Could you check a few things on this model? Use its own coordinates, in mm. A direction names the side the tool comes from. Round coordinates to 2 decimals unless told otherwise and drop trailing zeros. Write each loop counter-clockwise with the first axis right and the second up, starting at its lowest first coordinate (ties: lowest second). Pieces come first, ordered by that corner, then holes. Notation, with made-up numbers: (-31, -19) -> (-10, -19) arc R5 ccw to (-10, -15) -> close; hole circle Ø10 at (-38.75, 9). An arc over 180 degrees is marked (long way). Answer as CSV lines item,"result". Start each with the question number.
Q1. If we mould it in two halves opening along Z, with no side actions, what happens to faces 5 (the flat face through (42.99, -4.83, -6.68)), 6 (the cylindrical face through (8.33, 2.18, 22.03)), 7 (the flat face through (20.1, 3, 0))? For each: pulls with the +Z half, pulls with the -Z half, needs draft (parallel to the pull), parting line crosses it, or undercut.
Q2. Will these pins go through, and if not, where does the flat tip stop? pin 1 Ø3.5 at (x, y) = (8.9, 4) entering from -Z; pin 2 Ø3 at (x, z) = (55.5, 9) entering from +Y; pin 3 Ø3 at (y, z) = (21.51, 23.7) entering from -X.
Q3. Imagine slicing it at B-B on z = -16. Please give me the cut outline in (x, y), and give its area (3 significant figures).
Q4. Imagine slicing it at D-D on z = 35.2. Please give me the cut outline in (x, y).
Q5. Imagine slicing it at A-A on x = -5.6. Please give me the cut outline in (y, z).
Q6. For faces 1 (the flat face through (52.07, -2.02, 25.92)), 2 (the flat face through (0, 3, 20.1)), 3 (the cylindrical face through (71.44, -1.43, 25.05)), 4 (the flat face through (-23.9, 3, 0)), which set-ups out of +Z, -Z, +X, -X, +Y, -Y let a thin tool reach every point of the face, with its end or its side?
Q7. Imagine slicing it at C-C on y = 16.5. Please give me the cut outline in (x, z).
Q8. If I drill on line 1 (Y direction, x = 71, z = 46.7); line 2 (X direction, y = 2.5, z = 23); line 3 (Z direction, x = 20, y = 3.5), over which ranges is the centre line in solid material (lowest first)? Write a range as [from, to].
from build123d import *

# Parameters (mm, degrees)
SKETCH1_W            = 47.8
SKETCH1_H            = 47.8
SKETCH1_W_2          = 40.2
SKETCH1_H_2          = 40.2
BOSS_EXTRUDE1_DEPTH  = 6
CUT_EXTRUDE4_REACH   = 55.778
SKETCH6_R            = 1.35
CUT_EXTRUDE5_REACH   = 55.778
SKETCH7_R            = 1.35
SKETCH8_R            = 1.35
CUT_EXTRUDE6_DEPTH   = 54.777783517
SKETCH11_W           = 5
SKETCH11_H           = 28
SKETCH11_W_2         = 47.8
SKETCH11_H_2         = 47.8
SKETCH11_R           = 1.65
BOSS_EXTRUDE8_DEPTH  = 8
CUT_EXTRUDE7_DEPTH   = 105.25363303
SKETCH12_W           = 28
SKETCH12_H           = 28
SKETCH12_R           = 11.15
SKETCH12_R_2         = 1.35
SKETCH12_R_3         = 8.5
BOSS_EXTRUDE9_DEPTH  = 5
BOSS_EXTRUDE10_START = -2
SKETCH12_3_R         = 8.5
BOSS_EXTRUDE10_DEPTH = 3
SKETCH14_R           = 2.15
BOSS_EXTRUDE11_DEPTH = 8
SKETCH14_3_R         = 2.15
CUT_EXTRUDE8_DEPTH   = 10


with BuildPart() as part:
    # Sketch1 → Boss-Extrude1 (new body)
    with BuildSketch(Plane(origin=(0, 0, 0), x_dir=(1, 0, 0), z_dir=(0, 1, 0))):
        Rectangle(SKETCH1_W, SKETCH1_H)
        Rectangle(SKETCH1_W_2, SKETCH1_H_2, mode=Mode.SUBTRACT)
    extrude(amount=BOSS_EXTRUDE1_DEPTH)

    # Sketch6 → Cut-Extrude4 (cut, up to next)
    with BuildSketch(Plane(origin=(0, 0, -23.9), x_dir=(-1, 0, 0), z_dir=(0, 0, -1)), mode=Mode.PRIVATE) as cut_extrude4_sk1:
        with Locations((-8.9, 4)):
            Circle(SKETCH6_R)
    cut_extrude4_tool1 = extrude(cut_extrude4_sk1.sketch, amount=-CUT_EXTRUDE4_REACH, mode=Mode.PRIVATE) & part.part
    # Sketch6 → Cut-Extrude4 (cut, up to next)
    with BuildSketch(Plane(origin=(0, 0, -23.9), x_dir=(-1, 0, 0), z_dir=(0, 0, -1)), mode=Mode.PRIVATE) as cut_extrude4_sk2:
        with Locations((8.9, 4)):
            Circle(SKETCH6_R)
    cut_extrude4_tool2 = extrude(cut_extrude4_sk2.sketch, amount=-CUT_EXTRUDE4_REACH, mode=Mode.PRIVATE) & part.part
    add(cut_extrude4_tool1.solids().sort_by_distance((8.9, 4, -23.9))[0], mode=Mode.SUBTRACT)
    add(cut_extrude4_tool2.solids().sort_by_distance((-8.9, 4, -23.9))[0], mode=Mode.SUBTRACT)

    # Sketch7 → Cut-Extrude5 (cut, up to next)
    with BuildSketch(Plane.XY.offset(23.9), mode=Mode.PRIVATE) as cut_extrude5_sk1:
        with Locations((9.4, 3)):
            Circle(SKETCH7_R)
    cut_extrude5_tool1 = extrude(cut_extrude5_sk1.sketch, amount=-CUT_EXTRUDE5_REACH, mode=Mode.PRIVATE) & part.part
    # Sketch7 → Cut-Extrude5 (cut, up to next)
    with BuildSketch(Plane.XY.offset(23.9), mode=Mode.PRIVATE) as cut_extrude5_sk2:
        with Locations((-5.6, 3)):
            Circle(SKETCH7_R)
    cut_extrude5_tool2 = extrude(cut_extrude5_sk2.sketch, amount=-CUT_EXTRUDE5_REACH, mode=Mode.PRIVATE) & part.part
    add(cut_extrude5_tool1.solids().sort_by_distance((9.4, 3, 23.9))[0], mode=Mode.SUBTRACT)
    add(cut_extrude5_tool2.solids().sort_by_distance((-5.6, 3, 23.9))[0], mode=Mode.SUBTRACT)

    # Sketch8 → Cut-Extrude6 (cut, through all)
    with BuildSketch(Plane(origin=(23.9, 0, 0), x_dir=(0, 0, -1), z_dir=(1, 0, 0))):
        with Locations((-5.9, 4)):
            Circle(SKETCH8_R)
        with Locations(Location((5.9, 4, 0), (0, 0, 180))):
            Circle(SKETCH8_R)
    extrude(amount=-CUT_EXTRUDE6_DEPTH, mode=Mode.SUBTRACT)

    # Sketch11 → Boss-Extrude8 (add)
    # profile 1 of 3: a face of its own
    with BuildSketch(Plane(origin=(0, 0, 0), x_dir=(1, 0, 0), z_dir=(0, 1, 0))):
        Polygon((73.9, -21.2), (68.9, -21.2), (68.9, -49.2), (-23.9, -23.9), (23.9, -23.9), (23.9, 23.9), align=None)
    # profile 2 of 3: a face of its own
    with BuildSketch(Plane(origin=(0, 0, 0), x_dir=(1, 0, 0), z_dir=(0, 1, 0))):
        with Locations((71.4, -35.2)):
            Rectangle(SKETCH11_W, SKETCH11_H)
    # profile 3 of 3: a face of its own
    with BuildSketch(Plane(origin=(0, 0, 0), x_dir=(1, 0, 0), z_dir=(0, 1, 0))):
        Rectangle(SKETCH11_W_2, SKETCH11_H_2)
        with Locations(Location((-16, -16, 0), (0, 0, 270))):
            Circle(SKETCH11_R, mode=Mode.SUBTRACT)
        with Locations(Location((16, -16, 0), (0, 0, 270))):
            Circle(SKETCH11_R, mode=Mode.SUBTRACT)
        with Locations(Location((16, 16, 0), (0, 0, 270))):
            Circle(SKETCH11_R, mode=Mode.SUBTRACT)
        with Locations(Location((-16, 16, 0), (0, 0, 270))):
            Circle(SKETCH11_R, mode=Mode.SUBTRACT)
    extrude(amount=-BOSS_EXTRUDE8_DEPTH)

    # Sketch13 → Cut-Extrude7 (cut, through all)
    with BuildSketch(Plane.XY.offset(49.2)):
        Polygon((73.9, -3.987183479), (64.114380232, -3.987183479), (28.73812358, 1.78739259), (73.9, 1.78739259), align=None)
    extrude(amount=-CUT_EXTRUDE7_DEPTH, mode=Mode.SUBTRACT)

    # Sketch12 → Boss-Extrude9 (add)
    # profile 1 of 2: a face of its own
    with BuildSketch(Plane(origin=(73.9, 0, 0), x_dir=(0, 0, -1), z_dir=(1, 0, 0))):
        with Locations((-35.2, 10.012816521)):
            Rectangle(SKETCH12_W, SKETCH12_H)
        with Locations((-35.2, 10.012816521)):
            Circle(SKETCH12_R, mode=Mode.SUBTRACT)
        with Locations((-46.7, 21.512816521)):
            Circle(SKETCH12_R_2, mode=Mode.SUBTRACT)
        with Locations((-23.7, 21.512816521)):
            Circle(SKETCH12_R_2, mode=Mode.SUBTRACT)
        with Locations((-23.7, -1.487183479)):
            Circle(SKETCH12_R_2, mode=Mode.SUBTRACT)
        with Locations((-46.7, -1.487183479)):
            Circle(SKETCH12_R_2, mode=Mode.SUBTRACT)
    # profile 2 of 2: a face of its own
    with BuildSketch(Plane(origin=(73.9, 0, 0), x_dir=(0, 0, -1), z_dir=(1, 0, 0))):
        with Locations((-35.2, 10.012816521)):
            Circle(SKETCH12_R_3)
    extrude(amount=-BOSS_EXTRUDE9_DEPTH)


with BuildPart() as boss_extrude9_kept_piece:
    # of the separate pieces the step leaves, the one the design keeps (boss_extrude9_pieces_kept)
    add(part.part.solids().sort_by_distance((-23.9, 6, -23.9))[0])

    # Sketch12<3> → Boss-Extrude10 (add)
    # profile 1 of 2: a face of its own
    with BuildSketch(Plane(origin=(73.9, 0, 0), x_dir=(0, 0, -1), z_dir=(1, 0, 0)).offset(BOSS_EXTRUDE10_START)):
        with BuildLine():
            Line((-40.1057115, 0), (-30.2942885, 0))
            ThreePointArc((-30.2942885, 0), (-25.738996268, 4.112654795), (-24.05, 10.012816521))
            ThreePointArc((-24.05, 10.012816521), (-41.100161726, 19.473820253), (-40.1057115, 0))
        make_face()
        with Locations((-35.2, 10.012816521)):
            Circle(SKETCH12_3_R, mode=Mode.SUBTRACT)
    # profile 2 of 2: a face of its own
    with BuildSketch(Plane(origin=(73.9, 0, 0), x_dir=(0, 0, -1), z_dir=(1, 0, 0)).offset(BOSS_EXTRUDE10_START)):
        with BuildLine():
            ThreePointArc((-40.1057115, 0), (-35.2, -1.137183479), (-30.2942885, 0))
            Line((-30.2942885, 0), (-40.1057115, 0))
        make_face()
    extrude(amount=-BOSS_EXTRUDE10_DEPTH)

    # Sketch14 → Boss-Extrude11 (add)
    # profile 1 of 4: a face of its own
    with BuildSketch(Plane.XZ.offset(8)):
        with Locations((-24, -5)):
            Circle(SKETCH14_R)
    # profile 2 of 4: a face of its own
    with BuildSketch(Plane.XZ.offset(8)):
        Polygon((-23.9, 23.9), (-40.851983798, 4), (-30.045704848, -43.045704848), (14.045704848, -43.045704848), (23.9, -23.9), (-23.9, -23.9), align=None)
        with Locations(Location((-33, 4, 0), (0, 0, 270))):
            Circle(SKETCH14_R, mode=Mode.SUBTRACT)
        with Locations(Location((8, -37, 0), (0, 0, 270))):
            Circle(SKETCH14_R, mode=Mode.SUBTRACT)
        with Locations(Location((-24, -37, 0), (0, 0, 270))):
            Circle(SKETCH14_R, mode=Mode.SUBTRACT)
    # profile 3 of 4: a face of its own
    with BuildSketch(Plane.XZ.offset(8)):
        with BuildLine():
            ThreePointArc((-23.9, -2.852326841), (-26.15, -5), (-23.9, -7.147673159))
            Line((-23.9, -7.147673159), (-23.9, -2.852326841))
        make_face()
    # profile 4 of 4: a face of its own
    with BuildSketch(Plane.XZ.offset(8)):
        with BuildLine():
            Line((-23.9, -2.852326841), (-23.9, -7.147673159))
            ThreePointArc((-23.9, -7.147673159), (-22.444766899, -6.484503284), (-21.85, -5))
            ThreePointArc((-21.85, -5), (-22.444766899, -3.515496716), (-23.9, -2.852326841))
        make_face()
    extrude(amount=-BOSS_EXTRUDE11_DEPTH)

    # Sketch14<3> → Cut-Extrude8 (cut)
    with BuildSketch(Plane.XZ.offset(8)):
        with Locations(Location((29.5, 16.5, 0), (0, 0, 270))):
            Circle(SKETCH14_3_R)
    extrude(amount=-CUT_EXTRUDE8_DEPTH, mode=Mode.SUBTRACT)


solid = boss_extrude9_kept_piece.part
Checks:
1,face 5,"pulls with the -Z half"
1,face 6,"needs draft"
1,face 7,"undercut"
2,pin 1,"z = -23.9"
2,pin 2,"y = -2.34"
2,pin 3,"x = 68.9"
3,outline,"(-36.26, -8) -> (-17.65, -8) -> (-17.65, 0) -> (-20.1, 0) -> (-20.1, 6) -> (-23.9, 6) -> (-23.9, 0) -> (-36.26, 0) -> close; (-14.35, -8) -> (14.35, -8) -> (14.35, 0) -> (-14.35, 0) -> close; (17.65, -8) -> (32.66, -8) -> (32.66, 0) -> (23.9, 0) -> (23.9, 6) -> (20.1, 6) -> (20.1, 0) -> (17.65, 0) -> close"
3,area,"544 mm^2"
4,outline,"(17.55, -8) -> (73.9, -8) -> (73.9, -1.14) -> (71.9, -1.14) -> (71.9, 1.51) -> (68.9, 1.51) -> (68.9, -3.99) -> (64.11, -3.99) -> (39.69, 0) -> (17.55, 0) -> close; (68.9, 18.51) -> (71.9, 18.51) -> (71.9, 21.16) -> (73.9, 21.16) -> (73.9, 24.01) -> (68.9, 24.01) -> close"
5,outline,"(-8, -43.05) -> (0, -43.05) -> (0, -23.9) -> (6, -23.9) -> (6, -20.1) -> (0, -20.1) -> (0, 20.1) -> (1.65, 20.1) -> (1.65, 23.9) -> (0, 23.9) -> (0, 28.89) -> (-8, 28.89) -> close; (4.35, 20.1) -> (6, 20.1) -> (6, 23.9) -> (4.35, 23.9) -> close"
6,face 1,"+Z, -Z, +Y"
6,face 2,"+Y"
6,face 3,"+X"
6,face 4,"+Z, -Z, -X, +Y"
7,outline,"(68.9, 21.2) -> (73.9, 21.2) -> (73.9, 26.13) -> (71.9, 26.13) -> (71.9, 29.71) -> (68.9, 29.71) -> close; (68.9, 40.69) -> (71.9, 40.69) -> (71.9, 44.27) -> (73.9, 44.27) -> (73.9, 49.2) -> (68.9, 49.2) -> close"
8,line 1,"[-8, -2.84], [-0.14, 20.16], [22.86, 24.01]"
8,line 2,"[-23.9, -6.85], [-4.35, 8.15], [10.65, 23.9], [68.9, 73.9]"
8,line 3,"[-23.9, -20.1], [20.1, 23.9]"
